For this review, use the dimensioned drawing (mm, ordinates from the lowest corner) and the shaded views. A direction names the side the tool comes from. Give positions to 0.01 mm unless a question says otherwise; leave off trailing zeros. Order: outer loops, then holes, each group sorted by start corner. A loop starts at its lowest first (then second) coordinate and runs counter-clockwise, first axis right, second up.
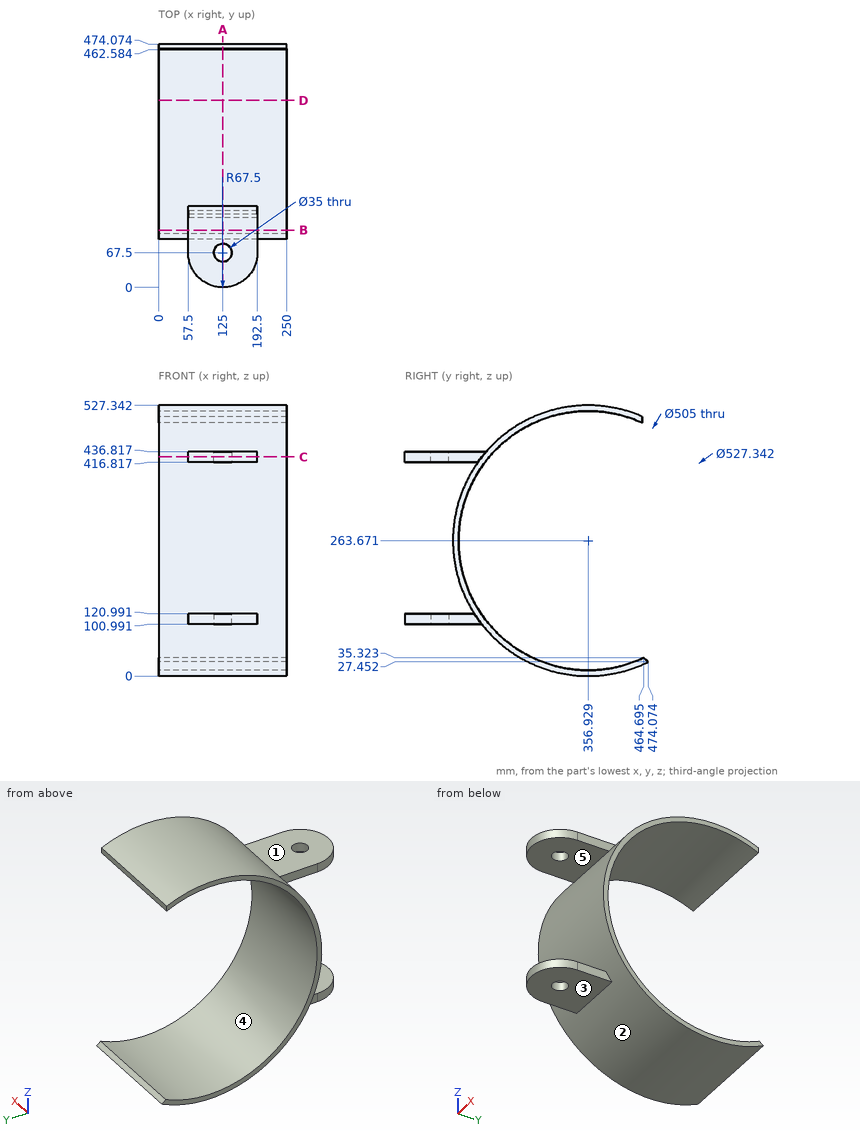
1. Take a section at C-C (z = 427). State the section outline as (x, y) points, then the cut area to 3 significant figures.
Recorded:
outline: (0, 149.94) - (57.5, 149.94) - (57.5, 67.5) arc R67.5 ccw to (192.5, 67.5) - (192.5, 149.94) - (250, 149.94) - (250, 164.37) - (0, 164.37) - close; hole circle Ø35 at (125, 67.5)
area: 20,900 mm2
2. For line 1 along X through (y, z) = (67.5, 113); line 2 along Z through (x, y) = (80, 66.5); line 3 along Y through (x, z) = (125, 421) (1 decimal), list the stretches that pass through material, from the lowest coordinate up.
Recorded:
line 1: x = 57.5 to 107.5, 142.5 to 192.5
line 2: z = 100.99 to 120.99, 416.82 to 436.82
line 3: y = 0 to 50, 85 to 159.4
3. Take a section at A-A (x = 125). State the section outline as (y, z) points (1 decimal).
Recorded:
outline: (0, 101) - (50, 101) - (50, 121) - (0, 121) - close; (0, 416.8) - (50, 416.8) - (50, 436.8) - (0, 436.8) - close; (85, 101) - (149.4, 101) arc R263.7 ccw to (474.1, 27.5) - (464.7, 35.3) arc R252.5 cw (long way) to (462.6, 493) - (462.6, 505.2) arc R263.7 ccw to (158.1, 436.8) - (85, 436.8) - (85, 416.8) - (142.3, 416.8) arc R263.7 ccw to (135.2, 121) - (85, 121) - close
4. Machinability: for the marked faces 4 and 5, which of the approach directions +Z, -Z, +X, -X, +Y, -Y give a long, thin tool a straight path to every point of the face, cutting with its end or side? Answer none if there is none.
Recorded:
face 4: +X, -X
face 5: +X, -X, -Y
5. For pin 1 (5 mm diameter, centred on x = 153, y = 111, fed in from +Z); pin 2 (16 mm diameter, centred on y = 118.5, z = 425.5, fed in from -X); pin 3 (10 mm diameter, centred on y = 99.5, z = 114, fed in from +X), all flat-tipped, find the tip position at first contact; note any pin that passes through.
Recorded:
pin 1: stops at z = 436.82
pin 2: stops at x = 57.5
pin 3: stops at x = 192.5
6. Take a section at B-B (y = 111.5). State the section outline as (x, z) points (1 decimal).
Recorded:
outline: (0, 167.3) - (250, 167.3) - (250, 204.3) - (0, 204.3) - close; (0, 323) - (250, 323) - (250, 360) - (0, 360) - close; (57.5, 101) - (192.5, 101) - (192.5, 121) - (57.5, 121) - close; (57.5, 416.8) - (192.5, 416.8) - (192.5, 436.8) - (57.5, 436.8) - close
7. Take a section at D-D (y = 364). State the section outline as (x, z) points (1 decimal), then the cut area to 3 significant figures.
Recorded:
outline: (0, 0.1) - (250, 0.1) - (250, 11.3) - (0, 11.3) - close; (0, 516.1) - (250, 516.1) - (250, 527.2) - (0, 527.2) - close
area: 5,590 mm2
8. Draft analysis for pull direction Z (two halves, no side actions). For the marked faces 1, 2 and 3, state which applies: pulls with the +Z half, pulls with the -Z half, needs draft (parallel to the pull), parting line crosses it, or undercut.
Recorded:
face 1: pulls with the +Z half
face 2: undercut
face 3: pulls with the -Z half
